Autodesk Inventor part; units mm, degrees
ref_plane "Work Plane1" through (0, 0, 7) normal (0, 0, -1) x (-1, 0, 0)
ref_plane "Work Plane2" through (8.175, 0, 0) normal (1, 0, 0) x (0, 1, 0)
ref_plane "XZ Plane" through (0, 0, 0) normal (0, 1, 0) x (-1, 0, 0)
sketch "Sketch1" plane through (0, 0, 0) normal (0, 0, 1) x (1, 0, 0)
  circle A0 centre (0, 0) radius 20
  circle A1 centre (0, 0) radius 25
  circle A2 centre (0, 0) radius 3.175
  circle A3 centre (0, 0) radius 8.175
  dimension "d18" = 6.35
  dimension "d19" = 16.35
  dimension "d40" = 40
  dimension "d41" = 5
extrude "Extrusion1" add sketch "Sketch1" along normal blind 14 contours A0 | A2 | A3
extrude "Extrusion2" add sketch "Sketch1" along normal blind 2 contours A1
sketch "Sketch2" plane through (0, 0, 14) normal (0, 0, 1) x (1, 0, 0)
  circle A0 centre (0, 0) radius 20
  circle A1 centre (0, 0) radius 25
extrude "Extrusion3" add sketch "Sketch2" against normal blind 2
ref_plane "Work Plane1" through (0, 0, 7) normal (0, 0, -1) x (-1, 0, 0)
extrude "Extrusion5" cut sketch "Sketch1" along normal up to surface (14 mm away) contours A2
extrude "Extrusion6" add sketch "Sketch1" against normal blind 14 contours A3
ref_plane "Work Plane2" through (8.175, 0, 0) normal (1, 0, 0) x (0, 1, 0)
sketch "Sketch9" plane through (0, 0, 7) normal (0, 0, -1) x (-1, 0, 0)
  circle A0 centre (0, 0) radius 20
  line L0 (0, -20) -> (0, -25) construction
  circle A1 centre (0, 0) radius 25
  arc A2 (0, -20) -> (0, -25) centre (7.5993, -22.5) ccw
  line L1 (0, -25) -> (-4.6567, -19.4503)
  circle A3 centre (0, 0) radius 20
  line L2 (17.3205, -10) -> (21.6506, -12.5) construction
  line L3 (21.6506, -12.5) -> (14.5161, -13.758)
  arc A4 (17.3205, -10) -> (21.6506, -12.5) centre (23.2852, -4.6688) ccw
  line L4 (17.3205, 10) -> (21.6506, 12.5) construction
  line L5 (21.6506, 12.5) -> (19.1728, 5.6923)
  arc A5 (17.3205, 10) -> (21.6506, 12.5) centre (15.6859, 17.8312) ccw
  line L6 (0, 20) -> (0, 25) construction
  line L7 (0, 25) -> (4.6567, 19.4503)
  arc A6 (0, 20) -> (0, 25) centre (-7.5993, 22.5) ccw
  line L8 (-17.3205, 10) -> (-21.6506, 12.5) construction
  line L9 (-21.6506, 12.5) -> (-14.5161, 13.758)
  arc A7 (-17.3205, 10) -> (-21.6506, 12.5) centre (-23.2852, 4.6688) ccw
  line L10 (-17.3205, -10) -> (-21.6506, -12.5) construction
  line L11 (-21.6506, -12.5) -> (-19.1728, -5.6923)
  arc A8 (-17.3205, -10) -> (-21.6506, -12.5) centre (-15.6859, -17.8312) ccw
  point P0 (0, -22.5)
  point P1 (19.4856, -11.25)
  point P2 (19.4856, 11.25)
  point P3 (0, 22.5)
  point P4 (-19.4856, 11.25)
  point P5 (-19.4856, -11.25)
  dimension "d58" = 8
  dimension "d59" = 40
  dimension "d62" = 360
extrude "Extrusion9" add sketch "Sketch9" along normal mid plane 4 contours A0 A5 L5 | A4 L3 A0 | A0 A6 L7 | A2 L1 A0 | L9 A0 A7 | L11 A0 A8
sketch "Sketch10" plane through (8.175, 0, 0) normal (1, 0, 0) x (0, 1, 0)
  line L0 (0, 0) -> (0, -14) construction
  line L1 (-8.175, -14) -> (8.175, -14) construction
  circle A0 centre (0, -7) radius 2.6543
  circle A1 centre (0, -7) radius 2.5273
  dimension "d66" = 5.3086
  dimension "d67" = 5.0546
extrude "Extrusion10" cut sketch "Sketch10" against normal blind 3.81 contours A1
loft "Loft1" cut profiles "Sketch10" section 2 edges at (4.365, -2.5273, -7) contours A0 | A1
hole "Hole2" at (8.175, 0, -7) direction (-1, 0, 0) diameter 3.797 end up to surface
properties part number "intermediateSpindle"
Model file for the job. Use its own axes, mm. A direction names the side the tool comes from. Coordinates: 2 decimals unless noted, no trailing zeros. Loops run counter-clockwise (first coordinate to the right, second up) from the corner with the lowest first, then second, coordinate; pieces in that order, holes last. Notation, with made-up numbers: M 1,85.25 L 14,85.25 A10 cw 14,100.25 Z; hole C 25,85 d5. An arc over 180 degrees is marked long. Use CSV: the item, a comma, the result in double quotes. Start each with the question number.
1. Two-plate mould, pull along Z, no slides. Class faces 1 (the flat face through (17, 12, 9)), 2 (the cylindrical face through (-3.17, -0.14, -0.2)), 3 (the flat face through (2.3, -22.26, 7.03)), 4 (the flat face through (0, -5, 14)): pulls with the +Z half, pulls with the -Z half, needs draft (parallel to the pull), parting line crosses it, or undercut.
2. Tool access for faces 5 (the flat face through (-19, 9, 5)), 6 (the flat face through (19, -9, 9)): list every direction of +Z, -Z, +X, -X, +Y, -Y with a clear straight run to the whole face (end or side of a thin tool).
3. Band-saw the part on A-A, the plane y = 0. List the corners of the cut face in (x, z) (1 decimal).
4. Band-saw the part on D-D, the plane y = 21. List the corners of the cut face in (x, z), then the cut area to 3 significant figures.
5. Flat gauge pins, fed straight in: pin 1 (2 mm diameter, centred on x = 18.5, y = 6, fed in from -Z); pin 2 (10 mm diameter, centred on y = -2, z = 8, fed in from -X); pin 3 (3 mm diameter, centred on y = 0, z = -7, fed in from +X); pin 4 (4 mm diameter, centred on y = -1, z = -6, fed in from +X) (3 decimals). Where does each tip first touch, or does it go through?
6. Probe probe 1 along Z at (x, y) = (18, -13.5); probe 2 along Z at (x, y) = (3.95, 0); probe 3 along Y at (x, z) = (0, 2.75) (3 decimals). List the from-to ranges inside material, lowest first. Write a range as [from, to].
7. Band-saw the part on B-B, the plane x = -18. List the corners of the cut face in (y, z).
8. Band-saw the part on C-C, the plane z = -1.25. List the corners of the cut face in (x, y) (3 decimals).
Entries:
1,face 1,"undercut"
1,face 2,"needs draft"
1,face 3,"undercut"
1,face 4,"pulls with the +Z half"
2,face 5,"-X, +Y"
2,face 6,"+X, -Y"
3,outline,"M -25,0 L -8.2,0 L -8.2,-14 L -3.2,-14 L -3.2,14 L -25,14 L -25,12 L -20,12 L -20,2 L -25,2 Z; M 3.2,-14 L 8.2,-14 L 8.2,-9.7 L 4.4,-9.5 L 4.4,-8.9 L 3.2,-8.9 Z; M 3.2,-5.1 L 4.4,-5.1 L 4.4,-4.5 L 8.2,-4.3 L 8.2,0 L 25,0 L 25,2 L 20,2 L 20,12 L 25,12 L 25,14 L 3.2,14 Z"
4,outline,"M -13.56,0 L 13.56,0 L 13.56,2 L -13.56,2 Z; M -13.56,12 L 13.56,12 L 13.56,14 L -13.56,14 Z; M -3.36,5 L -0.26,5 L -0.26,9 L -3.36,9 Z"
4,area,"121 mm2"
5,pin 1,"stops at z = 0"
5,pin 2,"stops at x = -25"
5,pin 3,"stops at x = -2.8"
5,pin 4,"stops at x = 8.175"
6,probe 1,"z = [0, 2], [12, 14]"
6,probe 2,"z = [-14, -8.9], [-5.1, 14]"
6,probe 3,"y = [-20, -3.175], [3.175, 20]"
7,outline,"M -17.35,0 L 17.35,0 L 17.35,2 L 8.72,2 L 8.72,5 L 10.17,5 L 10.17,9 L 8.72,9 L 8.72,12 L 17.35,12 L 17.35,14 L -17.35,14 L -17.35,12 L -8.72,12 L -8.72,2 L -17.35,2 Z; M -13.14,5 L -10.67,5 L -10.67,9 L -13.14,9 Z"
8,outline,"C 0,0 d16.35; hole C 0,0 d6.35"
